```python
from build123d import *

# Parameters (mm, degrees)
EXTRUDE_1_DEPTH = 20
SKETCH_4_R      = 1.5
EXTRUDE_2_DEPTH = 6
M3X0_5_1_D      = 2.5
M3X0_5_1_DEPTH  = 7.5
M3X0_5_1_TIP    = 0.751075774


with BuildPart() as part:
    # 草圖1 → 填料-伸長1 (new body)
    with BuildSketch(Plane.XY):
        Polygon((-1.443375673, 2.5), (-2.886751346, 0), (-1.443375673, -2.5), (1.443375673, -2.5), (2.886751346, 0), (1.443375673, 2.5), align=None)
    extrude(amount=EXTRUDE_1_DEPTH)

    # 草圖4 → 填料-伸長2 (add)
    with BuildSketch(Plane(origin=(0, 0, 0), x_dir=(-1, 0, 0), z_dir=(0, 0, -1))):
        Circle(SKETCH_4_R)
    extrude(amount=EXTRUDE_2_DEPTH)

    # M3x0.5 螺紋孔1
    with Locations(Plane.XY.offset(20)):
        with Locations((0, 0)):
            Hole(M3X0_5_1_D / 2, depth=M3X0_5_1_DEPTH)
            with Locations((0, 0, -(M3X0_5_1_DEPTH + M3X0_5_1_TIP / 2))):  # 118° drill point
                Cone(0, M3X0_5_1_D / 2, M3X0_5_1_TIP, mode=Mode.SUBTRACT)


solid = part.part
```
Could you check a few things on this model? Use its own coordinates, in mm. A direction names the side the tool comes from. Round coordinates to 2 decimals unless told otherwise and drop trailing zeros. Write each loop counter-clockwise with the first axis right and the second up, starting at its lowest first coordinate (ties: lowest second). Pieces come first, ordered by that corner, then holes. Notation, with made-up numbers: M -38,27.25 L -27,27.25 A13 cw -27,42.25 Z; hole C 71.5,17 d6. An arc over 180 degrees is marked long. Answer in a Markdown table with one row per item. Add a question column.
Q1. Will this pin go through, and if not, where does the flat tip stop? pin 1 Ø2 at (x, y) = (0, 0) entering from +Z.
Q2. If we mould it in two halves opening along X, with no side actions, what happens to faces 4 (the flat face through (-2.175, -1.233, 9.86)), 5 (the conical face through (-0.05, -0.21, 11.88)), 6 (the flat face through (2.175, 1.233, 9.86))? For each: +X half, -X half, draft (parallel to the pull), parting line (faces both ways), or undercut.
Q3. If I drill on line 1 (Y direction, x = 0, z = 16.5); line 2 (Z direction, x = -1.7, y = -0.55); line 3 (Y direction, x = -0.75, z = 13.5), over which ranges is the centre line in solid material (lowest first)? Write a range as from..to.
Q4. Imagine slicing it at C-C (y = 1.8). Please give me the cut outline in (x, z).
Q5. On a 3-axis mill with a long thin cutter (end or side, diameter ignored), from which of +Z, -Z, +X, -X, +Y, -Y can I reach the whole of each face in a straight line? I mean faces 1 (the cylindrical face through (0.27, -1.22, 16.2)), 2 (the flat face through (0, 0, -6)), 3 (the cylindrical face through (1.5, 0.07, -2.96)). Say none if no direction works.
Q6. Imagine slicing it at D-D (x = 2.2). Please give me the cut outline in (y, z).
Q7. Imagine slicing it at A-A (z = 13.25). Please give me the cut outline in (x, y).
Q8. Imagine slicing it at B-B (z = 10.5). Please give me the cut outline in (x, y), then the cut area to 3 significant figures.
Values:
| question | item | result |
|---|---|---|
| 1 | pin 1 | z = 12.35 |
| 2 | face 4 | -X half |
| 2 | face 5 | undercut |
| 2 | face 6 | +X half |
| 3 | line 1 | -2.5..-1.25, 1.25..2.5 |
| 3 | line 2 | 0..20 |
| 3 | line 3 | -2.5..-1, 1..2.5 |
| 4 | outline | M -1.85,0 L 1.85,0 L 1.85,20 L -1.85,20 Z |
| 5 | face 1 | +Z |
| 5 | face 2 | -Z, +X, -X, +Y, -Y |
| 5 | face 3 | -Z |
| 6 | outline | M -1.19,0 L 1.19,0 L 1.19,20 L -1.19,20 Z |
| 7 | outline | M -2.89,0 L -1.44,-2.5 L 1.44,-2.5 L 2.89,0 L 1.44,2.5 L -1.44,2.5 Z; hole C 0,0 d2.5 |
| 8 | outline | M -2.89,0 L -1.44,-2.5 L 1.44,-2.5 L 2.89,0 L 1.44,2.5 L -1.44,2.5 Z |
| 8 | area | 21.7 mm^2 |
